Input: part model. Units: mm. Frame: model coordinates. Face numbers are marked on the shaded views. A direction names the side the tool comes from. Give positions to 0.01 mm unless a question says otherwise; leave off trailing zeros. Order: outer loops, then holes, each group sorted by start corner. A loop starts at its lowest first (then second) coordinate and runs counter-clockwise, first axis right, second up. Notation, with made-up numbers: M 22.25,38.25 L 73.25,38.25 A17 cw 73.25,56.25 Z; hole C 31,17.5 d9. An arc over 180 degrees is marked long. Use a Markdown table: item, result.
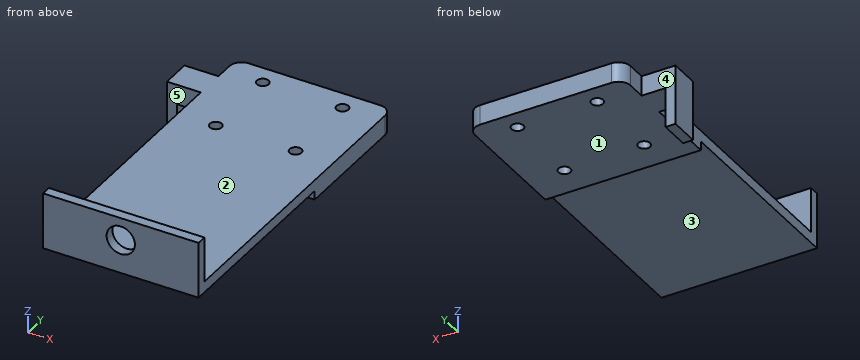
from build123d import *

# Parameters (mm, degrees)
CROQUIS1_R              = 3
SALIENTE_EXTRUIR1_DEPTH = 10
REDONDEO3_R             = 6
REDONDEO4_R             = 6
CROQUIS3_W              = 78
CROQUIS3_H              = 99
SALIENTE_EXTRUIR2_DEPTH = 5.5
CROQUIS4_W              = 78
CROQUIS4_H              = 22.679982155
SALIENTE_EXTRUIR3_DEPTH = 5
CROQUIS6_R              = 7.1
CORTAR_EXTRUIR1_DEPTH   = 40
CROQUIS7_W              = 20
CROQUIS7_H              = 15
SALIENTE_EXTRUIR4_DEPTH = 5


with BuildPart() as part:
    # Croquis1 → Saliente-Extruir1 (new body)
    with BuildSketch(Plane.XY):
        Polygon((0, 0), (78, 0), (78, -66), (0, -66), (0, -30.5), (-10, -30.5), (-17, -30.5), (-17, -15.5), (0, -15.5), align=None)
        with Locations((19, -10)):
            Circle(CROQUIS1_R, mode=Mode.SUBTRACT)
        with Locations((19, -50)):
            Circle(CROQUIS1_R, mode=Mode.SUBTRACT)
        with Locations(Location((59, -50, 0), (0, 0, 180))):
            Circle(CROQUIS1_R, mode=Mode.SUBTRACT)
        with Locations(Location((59, -10, 0), (0, 0, 180))):
            Circle(CROQUIS1_R, mode=Mode.SUBTRACT)
    extrude(amount=SALIENTE_EXTRUIR1_DEPTH)

    # Redondeo3
    redondeo3_edges = [part.edges().sort_by_distance(p)[0] for p in [
        (0, 0, 5),
    ]]
    fillet(redondeo3_edges, radius=REDONDEO3_R)

    # Redondeo4
    redondeo4_edges = [part.edges().sort_by_distance(p)[0] for p in [
        (78, 0, 5),
    ]]
    fillet(redondeo4_edges, radius=REDONDEO4_R)

    # Croquis3 → Saliente-Extruir2 (add)
    with BuildSketch(Plane.XY.offset(10)):
        with Locations((39, -115.5)):
            Rectangle(CROQUIS3_W, CROQUIS3_H)
    extrude(amount=-SALIENTE_EXTRUIR2_DEPTH)

    # Croquis4 → Saliente-Extruir3 (add)
    with BuildSketch(Plane.XZ.offset(165)):
        with Locations((39, 21.339991078)):
            Rectangle(CROQUIS4_W, CROQUIS4_H)
    extrude(amount=-SALIENTE_EXTRUIR3_DEPTH)

    # Croquis6 → Cortar-Extruir1 (cut)
    with BuildSketch(Plane(origin=(0, -160, 0), x_dir=(1, 0, 0), z_dir=(0, 1, 0))):
        with Locations(Location((39, -21.339991078, 0), (0, 0, 270))):
            Circle(CROQUIS6_R)
    extrude(amount=-CORTAR_EXTRUIR1_DEPTH, mode=Mode.SUBTRACT)

    # Croquis7 → Saliente-Extruir4 (add)
    with BuildSketch(Plane.ZY.offset(17)):
        with Locations((-10, -23)):
            Rectangle(CROQUIS7_W, CROQUIS7_H)
    extrude(amount=-SALIENTE_EXTRUIR4_DEPTH)


solid = part.part
1) Reachability of the marked faces 1, 2, 3, 4 and 5 from +Z, -Z, +X, -X, +Y, -Y: full face, straight path, thin tool, end or side. Return the list, or none.
Response values:
| item | result |
|---|---|
| face 1 | -Z, +X, +Y, -Y |
| face 2 | +Z, +X, -X, +Y |
| face 3 | -Z, +X, -X, -Y |
| face 4 | +Z, -Z, -X, +Y |
| face 5 | +Z, -Z, -X, -Y |
2) Cut plane C-C on x = 39. Return loops of the section in (y, z), and give its area (3 significant figures).
Response values:
| item | result |
|---|---|
| outline | M -165,4.5 L -66,4.5 L -66,0 L 0,0 L 0,10 L -160,10 L -160,14.24 L -165,14.24 Z; M -165,28.44 L -160,28.44 L -160,32.68 L -165,32.68 Z |
| area | 1,250 mm² |
3) Cut plane A-A on x = 59. Return loops of the section in (y, z), and give its area (3 significant figures).
Response values:
| item | result |
|---|---|
| outline | M -165,4.5 L -66,4.5 L -66,0 L -53,0 L -53,10 L -160,10 L -160,32.68 L -165,32.68 Z; M -47,0 L -13,0 L -13,10 L -47,10 Z; M -7,0 L 0,0 L 0,10 L -7,10 Z |
| area | 1,200 mm² |
4) Cut plane D-D on z = 21.5. Return loops of the section in (x, y), and give its area (3 significant figures).
Response values:
| item | result |
|---|---|
| outline | M 0,-165 L 31.9,-165 L 31.9,-160 L 0,-160 Z; M 46.1,-165 L 78,-165 L 78,-160 L 46.1,-160 Z |
| area | 319 mm² |
5) First-contact query: pin 1 Ø3.5 at (x, y) = (19, -50) entering from +Z (3 decimals); pin 2 Ø4 at (x, y) = (28.5, -56.5) entering from +Z; pin 3 Ø8 at (x, z) = (-7, 1.5) entering from -Y; pin 4 Ø2 at (x, z) = (24, 1.5) entering from -Y. Flat tips, straight axial feed; report the tip coordinate or a pass-through.
Response values:
| item | result |
|---|---|
| pin 1 | passes through |
| pin 2 | stops at z = 10 |
| pin 3 | stops at y = -30.5 |
| pin 4 | stops at y = -66 |
6) Cut plane B-B on y = -50. Return loops of the section in (x, z), and give its area (3 significant figures).
Response values:
| item | result |
|---|---|
| outline | M 0,0 L 16,0 L 16,10 L 0,10 Z; M 22,0 L 56,0 L 56,10 L 22,10 Z; M 62,0 L 78,0 L 78,10 L 62,10 Z |
| area | 660 mm² |
7) Material intervals for line 1 (Y direction, x = 19, z = 7); line 2 (Z direction, x = 38, y = -42.5); line 3 (Y direction, x = 57, z = 15), sorted ascending. Write a range as from..to.
Response values:
| item | result |
|---|---|
| line 1 | y = -165..-53, -47..-13, -7..0 |
| line 2 | z = 0..10 |
| line 3 | y = -165..-160 |
